Could you check a few things on this model? Use its own coordinates, in mm. Face numbers are marked on the shaded views. A direction names the side the tool comes from. Give positions to 0.01 mm unless a question says otherwise; leave off trailing zeros. Write each loop counter-clockwise with the first axis right and the second up, starting at its lowest first coordinate (ties: lowest second). Pieces come first, ordered by that corner, then holes. Notation, with made-up numbers: (68, 67) - (107, 67) arc R19 ccw to (107, 92) - close; hole circle Ø10 at (-4, 38). An arc over 180 degrees is marked (long way). Write item = value, one per line.
from build123d import *

# Parameters (mm, degrees)
BOSS_EXTRUDE3_DEPTH = 25.4
CUT_EXTRUDE2_DEPTH  = 94.85387731
CUT_EXTRUDE3_START  = -22.86
CUT_EXTRUDE3_DEPTH  = 22.86
SKETCH8_R           = 10.7823
BOSS_EXTRUDE4_DEPTH = 22.86


with BuildPart() as part:
    # Sketch4 → Boss-Extrude3 (new body)
    with BuildSketch(Plane.XY):
        with BuildLine():
            Line((0, 0), (28.5877, 0))
            Line((28.5877, 0), (28.5877, -33.528))
            ThreePointArc((28.5877, -33.528), (39.37, -44.3103), (50.1523, -33.528))
            Line((50.1523, -33.528), (50.1523, 0))
            Line((50.1523, 0), (78.74, 0))
            Line((78.74, 0), (78.74, 34.036))
            Line((78.74, 34.036), (0, 34.036))
            Line((0, 34.036), (0, 0))
        make_face()
    extrude(amount=BOSS_EXTRUDE3_DEPTH)

    # Sketch5 → Cut-Extrude2 (cut, through all)
    with BuildSketch(Plane.XY.offset(25.4)):
        Polygon((47.498, 23.495), (56.388, 23.495), (56.388, 10.541), (22.352, 10.541), (22.352, 23.495), (31.242, 23.495), (31.242, 34.036), (47.498, 34.036), align=None)
    extrude(amount=-CUT_EXTRUDE2_DEPTH, mode=Mode.SUBTRACT)

    # Sketch7 → Cut-Extrude3 (cut)
    with BuildSketch(Plane.XY.offset(25.4).offset(CUT_EXTRUDE3_START)):
        with BuildLine():
            Line((28.5877, 0), (50.1523, 0))
            Line((50.1523, 0), (50.1523, -33.528))
            ThreePointArc((50.1523, -33.528), (39.37, -44.3103), (28.5877, -33.528))
            Line((28.5877, -33.528), (28.5877, 0))
        make_face()
    extrude(amount=CUT_EXTRUDE3_DEPTH, mode=Mode.SUBTRACT)

    # Sketch8 → Boss-Extrude4 (add)
    with BuildSketch(Plane.XY.offset(2.54)):
        with Locations((39.37, -33.528)):
            Circle(SKETCH8_R)
    extrude(amount=BOSS_EXTRUDE4_DEPTH)


solid = part.part
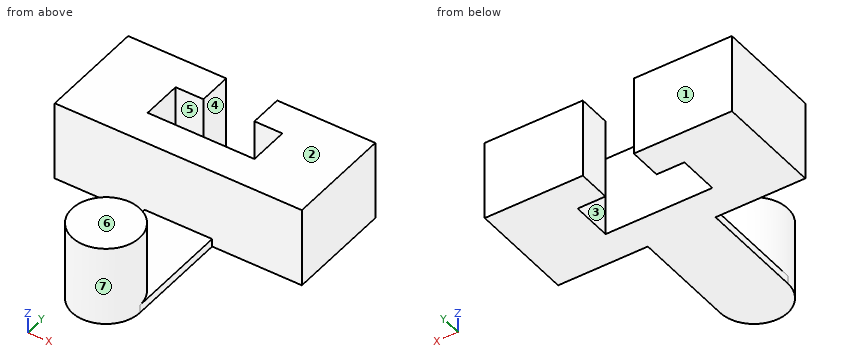
1. If we section it at A-A, the plane z = 4.25: Please give me the cut outline in (x, y) (3 decimals), and give its area (3 significant figures).
Filled sheet:
outline = (0, 0) - (78.74, 0) - (78.74, 34.036) - (47.498, 34.036) - (47.498, 23.495) - (56.388, 23.495) - (56.388, 10.541) - (22.352, 10.541) - (22.352, 23.495) - (31.242, 23.495) - (31.242, 34.036) - (0, 34.036) - close; circle Ø21.565 at (39.37, -33.528)
area = 2,430 mm2
2. For pin 1 (12 mm diameter, centred on x = 27.5, y = -31, fed in from -Z); pin 2 (3 mm diameter, centred on y = -10.5, z = 1, fed in from -X); pin 3 (10 mm diameter, centred on x = 27.5, z = 6.5, fed in from -Y); pin 4 (8 mm diameter, centred on y = -21.5, z = 10, fed in from +X), each with a flat end and sliding along its axis, tell me the tip position at first contact or that it passes through.
Filled sheet:
pin_1 = 0
pin_2 = 28.59
pin_3 = -41.84
pin_4 = 46.57
3. I need wall thicknesses on line 1 (Y direction, x = 51, z = 9.5) (3 decimals); line 2 (X direction, y = 11, z = 23.5); line 3 (Y direction, x = 29.5, z = 17.25) (3 decimals). Which ranges of each line are inside material? Lowest first, please.
Filled sheet:
line_1 = 0 to 10.541, 23.495 to 34.036
line_2 = 0 to 22.35, 56.39 to 78.74
line_3 = -37.869 to -29.187, 0 to 10.541, 23.495 to 34.036
4. If we section it at B-B, the plane y = 20.5: Please give me the cut outline in (x, z).
Filled sheet:
outline = (0, 0) - (22.35, 0) - (22.35, 25.4) - (0, 25.4) - close; (56.39, 0) - (78.74, 0) - (78.74, 25.4) - (56.39, 25.4) - close
5. Thinking about a two-plate mould opening in Y: for the marked faces 1, 2 and 3, which applies, pulls with the +Y half, pulls with the -Y half, needs draft (parallel to the pull), parting line crosses it, or undercut?
Filled sheet:
face_1 = pulls with the +Y half
face_2 = needs draft
face_3 = undercut
6. If we section it at C-C, the plane x = 39.37: Please give me the cut outline in (y, z).
Filled sheet:
outline = (-44.31, 0) - (10.54, 0) - (10.54, 25.4) - (0, 25.4) - (0, 2.54) - (-22.75, 2.54) - (-22.75, 25.4) - (-44.31, 25.4) - close
7. If we section it at D-D, the plane y = -13.5: Please give me the cut outline in (x, z), and give its area (3 significant figures).
Filled sheet:
outline = (28.59, 0) - (50.15, 0) - (50.15, 2.54) - (28.59, 2.54) - close
area = 54.8 mm2
8. Which directions (+Z, -Z, +X, -X, +Y, -Y) give clear straight access to the entire face, cutting with the end or side of a thin tool? Please do the marked faces 4, 5, 6 and 7.
Filled sheet:
face_4 = +Z, -Z, +Y
face_5 = +Z, -Z
face_6 = +Z, +X, -X, +Y, -Y
face_7 = +Z
